```python
from build123d import *

# Parameters (mm, degrees)
SKETCH1_R           = 60
BOSS_EXTRUDE1_DEPTH = 4
SKETCH2_R           = 2
SKETCH2_R_2         = 20
CUT_EXTRUDE1_DEPTH  = 4
SKETCH3_R           = 2
CUT_EXTRUDE2_DEPTH  = 4
SKETCH4_R           = 2
CUT_EXTRUDE3_DEPTH  = 4


with BuildPart() as part:
    # Sketch1 → Boss-Extrude1 (new body)
    with BuildSketch(Plane(origin=(0, 0, 0), x_dir=(1, 0, 0), z_dir=(0, 1, 0))):
        with BuildLine():
            Line((-219, 50), (-219, -100))
            Line((-219, -100), (-261, -100))
            Line((-261, -100), (-261, -120))
            Line((-261, -120), (-150, -160))
            Line((-150, -160), (150, -160))
            Line((150, -160), (261, -120))
            Line((261, -120), (261, -100))
            Line((261, -100), (219, -100))
            Line((219, -100), (219, 50))
            Line((219, 50), (261, 50))
            Line((261, 50), (261, 160))
            Line((261, 160), (110, 331.658711753))
            ThreePointArc((110, 331.658711753), (0, 382.155640476), (-110, 331.658711753))
            Line((-110, 331.658711753), (-261, 160))
            Line((-261, 160), (-261, 50))
            Line((-261, 50), (-219, 50))
        make_face()
        with Locations(Location((0, 215, 0), (0, 0, 270))):
            Circle(SKETCH1_R, mode=Mode.SUBTRACT)
    extrude(amount=BOSS_EXTRUDE1_DEPTH)

    # Sketch2 → Cut-Extrude1 (cut)
    with BuildSketch(Plane(origin=(0, 4, 0), x_dir=(1, 0, 0), z_dir=(0, 1, 0))):
        with Locations(Location((-206.3, -25, 0), (0, 0, 270))):
            Circle(SKETCH2_R)
        with Locations(Location((-206.3, 5, 0), (0, 0, 270))):
            Circle(SKETCH2_R)
        with Locations(Location((-206.3, 35, 0), (0, 0, 270))):
            Circle(SKETCH2_R)
        with Locations(Location((-206.3, -55, 0), (0, 0, 270))):
            Circle(SKETCH2_R)
        with Locations(Location((-206.3, -85, 0), (0, 0, 270))):
            Circle(SKETCH2_R)
        with Locations(Location((206.3, -85, 0), (0, 0, 270))):
            Circle(SKETCH2_R)
        with Locations(Location((206.3, -55, 0), (0, 0, 270))):
            Circle(SKETCH2_R)
        with Locations(Location((206.3, 5, 0), (0, 0, 270))):
            Circle(SKETCH2_R)
        with Locations(Location((206.3, 35, 0), (0, 0, 270))):
            Circle(SKETCH2_R)
        with Locations(Location((206.3, -25, 0), (0, 0, 270))):
            Circle(SKETCH2_R)
        with Locations(Location((0, -100, 0), (0, 0, 270))):
            Circle(SKETCH2_R_2)
    extrude(amount=-CUT_EXTRUDE1_DEPTH, mode=Mode.SUBTRACT)

    # Sketch3 → Cut-Extrude2 (cut)
    with BuildSketch(Plane(origin=(0, 4, 0), x_dir=(1, 0, 0), z_dir=(0, 1, 0))):
        with Locations(Location((0, 318.958711753, 0), (0, 0, 270))):
            Circle(SKETCH3_R)
        with Locations(Location((30, 318.958711753, 0), (0, 0, 270))):
            Circle(SKETCH3_R)
        with Locations(Location((60, 318.958711753, 0), (0, 0, 270))):
            Circle(SKETCH3_R)
        with Locations(Location((90, 318.958711753, 0), (0, 0, 270))):
            Circle(SKETCH3_R)
        with Locations(Location((-30, 318.958711753, 0), (0, 0, 270))):
            Circle(SKETCH3_R)
        with Locations(Location((-60, 318.958711753, 0), (0, 0, 270))):
            Circle(SKETCH3_R)
        with Locations(Location((-90, 318.958711753, 0), (0, 0, 270))):
            Circle(SKETCH3_R)
        with Locations(Location((0, -147.3, 0), (0, 0, 270))):
            Circle(SKETCH3_R)
        with Locations(Location((30, -147.3, 0), (0, 0, 270))):
            Circle(SKETCH3_R)
        with Locations(Location((60, -147.3, 0), (0, 0, 270))):
            Circle(SKETCH3_R)
        with Locations(Location((90, -147.3, 0), (0, 0, 270))):
            Circle(SKETCH3_R)
        with Locations(Location((-30, -147.3, 0), (0, 0, 270))):
            Circle(SKETCH3_R)
        with Locations(Location((-60, -147.3, 0), (0, 0, 270))):
            Circle(SKETCH3_R)
        with Locations(Location((-90, -147.3, 0), (0, 0, 270))):
            Circle(SKETCH3_R)
    extrude(amount=-CUT_EXTRUDE2_DEPTH, mode=Mode.SUBTRACT)

    # Sketch4 → Cut-Extrude3 (cut)
    with BuildSketch(Plane(origin=(0, 4, 0), x_dir=(1, 0, 0), z_dir=(0, 1, 0))):
        with Locations(Location((-20, -5, 0), (0, 0, 270))):
            Circle(SKETCH4_R)
        with Locations(Location((20, -5, 0), (0, 0, 270))):
            Circle(SKETCH4_R)
        with Locations(Location((20, -45, 0), (0, 0, 270))):
            Circle(SKETCH4_R)
        with Locations(Location((-20, -45, 0), (0, 0, 270))):
            Circle(SKETCH4_R)
    extrude(amount=-CUT_EXTRUDE3_DEPTH, mode=Mode.SUBTRACT)


solid = part.part
```
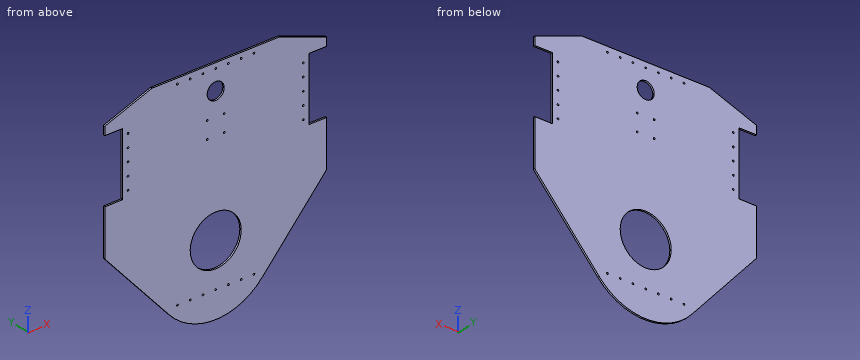
Geometry: final body of the model. Coordinates: model frame, mm. Round coordinates to 2 decimals unless told otherwise and drop trailing zeros. Order: outer loops, then holes, each group sorted by start corner. A loop starts at its lowest first (then second) coordinate and runs counter-clockwise, first axis right, second up. Notation, with made-up numbers: (-23.5, 73.25) - (22.5, 73.25) arc R19 cw to (22.5, 105.25) - close; hole circle Ø3 at (38, 57). An arc over 180 degrees is marked (long way). Write item = value, one per line. Start each with the question number.
Q1. Ray query, line 1 (X direction, y = 1.4, z = 5); line 2 (X direction, y = 2.7, z = 85); line 3 (X direction, y = 2.5, z = -240). Return the intervals inside material, ascending. Write a range as from..to.
Q2. Cut plane C-C on x = 157. Return the cut outline in (y, z), and give its area (3 significant figures).
Q3. Cut plane A-A on z = -254. Return the cut outline in (x, y).
Q4. Cut plane D-D on x = -130.5. Return the cut outline in (y, z), and give its area (3 significant figures).
Q5. Cut plane B-B on y = 3.15. Give the number of separate pieces and of enclosed holes in the cut face, and give its area (3 significant figures).
Q6. Pin query (flat end, axial travel): pin 1 (1.2 mm diameter, centred on y = 1.5, z = 37, fed in from -X); pin 2 (2 mm diameter, centred on x = 236, y = 2, fed in from +Z). Return the tip coordinate at first contact, or that it passes through.
Outcome:
q1.line_1 = -219..-22, -18..18, 22..219
q1.line_2 = -219..-208.3, -204.3..-13.23, 13.23..204.3, 208.3..219
q1.line_3 = -190.63..-54.54, 54.54..190.63
q2.outline = (0, -278.23) - (4, -278.23) - (4, 157.48) - (0, 157.48) - close
q2.area = 1,740 mm^2
q3.outline = (-178.31, 0) - (-45.6, 0) - (-45.6, 4) - (-178.31, 4) - close; (45.6, 0) - (178.31, 0) - (178.31, 4) - (45.6, 4) - close
q4.outline = (0, -308.35) - (4, -308.35) - (4, 160) - (0, 160) - close
q4.area = 1,870 mm^2
q5.separate_pieces = 1
q5.enclosed_holes = 30
q5.area = 208,000 mm^2
q6.pin_1 = -219
q6.pin_2 = 129.37
